The model under review builds one solid part; all positions refer to its coordinate system, in mm. A direction names the side the tool comes from. Round coordinates to 2 decimals unless told otherwise and drop trailing zeros. Order: outer loops, then holes, each group sorted by start corner. A loop starts at its lowest first (then second) coordinate and runs counter-clockwise, first axis right, second up. Notation, with made-up numbers: M -17.5,9 L 22.5,9 A15 ccw 22.5,30 Z; hole C -36,74.25 d4. An arc over 180 degrees is marked long. Use a Markdown table: item, result. Add a question column.
1. Consider section D-D on x = -50.5. State the section outline as (y, z) points, then the cut area to 3 significant figures.
2. To check wall thickness, follow probe 1 along Y at (x, z) = (0, 2.95); probe 2 along Z at (x, y) = (-38.5, -0.25); probe 3 along Y at (x, z) = (-8.5, 12). State the ranges of each line that lie inside material, in increasing order.
3. Consider section C-C on y = 3. State the section outline as (x, z) points, then the cut area to 3 significant figures.
4. Insertion check: P1, Ø4, axis at x = -46, y = -1, coming from the +Z side; P2, Ø1.2, axis at y = -1, z = 10, coming from the +X side; P3, Ø6, axis at x = -41, z = 12.5, coming from the -Y side. Each pin has a flat end and moves straight along its axis. Give the tip position at first contact, or say it passes through.
5. Consider section A-A on x = 0. State the section outline as (y, z) points.
6. The part is to be moulded in two halves that separate along Z. For faces 4 (the flat face through (0, -2, 12.6)), 5 (the flat face through (-33, 0, 6.3)), 6 (the cylindrical face through (-0.37, -1.66, 2.96)), 7 (the flat face through (-4.5, 0, 9)), say which applies: +Z half, -Z half, draft (parallel to the pull), parting line (faces both ways), or undercut.
7. For faces 1 (the flat face through (0, -2, 6)), 2 (the flat face through (-33, 0, 12.3)), 3 (the flat face through (-21, -2, 9)), list the 3-axis set-ups (+Z, -Z, +X, -X, +Y, -Y) from which the entire face can be reached by the end or side of a thin tool; tool diameter is ignored.
8. Consider section B-B on y = 0. State the section outline as (x, z) points.
from build123d import *

# Parameters (mm, degrees)
SKETCH_1_R           = 4
SKETCH_1_R_2         = 1.7
EXTRUDE_1_DEPTH      = 6
EXTRUDE_2_DEPTH      = 2
EXTRUDE_2_DEPTH_BACK = 2
SKETCH_3_R           = 1.7
EXTRUDE_3_DEPTH      = 3
EXTRUDE_3_DEPTH_BACK = 3


with BuildPart() as part:
    # Sketch 1 → Extrude 1 (new body)
    with BuildSketch(Plane.XY):
        Circle(SKETCH_1_R)
        Circle(SKETCH_1_R_2, mode=Mode.SUBTRACT)
    extrude_1 = extrude(amount=EXTRUDE_1_DEPTH)

    # Sketch 2 → Extrude 2 (add, two sides)
    with BuildSketch(Plane(origin=(0, 0, 0), x_dir=(1, 0, 0), z_dir=(0, 1, 0))) as extrude_2_sk:
        Polygon((-4, 0), (-10.5, -6), (-10.5, -12.6), (-4, -18.6), (-3, -18.6), (-3, -12.6), (-4, -12.6), (-4.5, -12.6), (-4.5, -6), (-4, -6), (-3, -6), (-3, 0), align=None)
    extrude(amount=EXTRUDE_2_DEPTH)
    extrude(extrude_2_sk.sketch, amount=-EXTRUDE_2_DEPTH_BACK)

    # Mirror 1: Extrude 1 across plane
    add(extrude_1.mirror(Plane(origin=(0, 0, 9.3), x_dir=(1, 0, 0), z_dir=(0, 0, -1))))

    # Sketch 3 → Extrude 3 (add, two sides)
    with BuildSketch(Plane(origin=(0, 0, 9.3), x_dir=(-1, 0, 0), z_dir=(0, 0, -1))) as extrude_3_sk:
        with BuildLine():
            Line((10.5, 2), (47.035898385, 2))
            ThreePointArc((47.035898385, 2), (54.5, 0), (47.035898385, -2))
            Line((47.035898385, -2), (10.5, -2))
            Line((10.5, -2), (10.5, 2))
        make_face()
        with Locations((50.5, 0)):
            Circle(SKETCH_3_R, mode=Mode.SUBTRACT)
    extrude(amount=EXTRUDE_3_DEPTH)
    extrude(extrude_3_sk.sketch, amount=-EXTRUDE_3_DEPTH_BACK)


solid = part.part
Answer block:
| question | item | result |
|---|---|---|
| 1 | outline | M -4,6.3 L -1.7,6.3 L -1.7,12.3 L -4,12.3 Z; M 1.7,6.3 L 4,6.3 L 4,12.3 L 1.7,12.3 Z |
| 1 | area | 27.6 mm^2 |
| 2 | probe 1 | -4 to -1.7, 1.7 to 4 |
| 2 | probe 2 | 6.3 to 12.3 |
| 2 | probe 3 | -2 to 2 |
| 3 | outline | M -53.15,6.3 L -47.85,6.3 L -47.85,12.3 L -53.15,12.3 Z; M -2.65,0 L 2.65,0 L 2.65,6 L -2.65,6 Z; M -2.65,12.6 L 2.65,12.6 L 2.65,18.6 L -2.65,18.6 Z |
| 3 | area | 95.2 mm^2 |
| 4 | P1 | z = 12.3 |
| 4 | P2 | x = -4.5 |
| 4 | P3 | y = -2 |
| 5 | outline | M -4,0 L -1.7,0 L -1.7,6 L -4,6 Z; M -4,12.6 L -1.7,12.6 L -1.7,18.6 L -4,18.6 Z; M 1.7,0 L 4,0 L 4,6 L 1.7,6 Z; M 1.7,12.6 L 4,12.6 L 4,18.6 L 1.7,18.6 Z |
| 6 | face 4 | undercut |
| 6 | face 5 | -Z half |
| 6 | face 6 | draft |
| 6 | face 7 | undercut |
| 7 | face 1 | +X, +Y, -Y |
| 7 | face 2 | +Z, -X, +Y, -Y |
| 7 | face 3 | +Z, -Z, -Y |
| 8 | outline | M -54.5,6.3 L -52.2,6.3 L -52.2,12.3 L -54.5,12.3 Z; M -48.8,6.3 L -10.5,6.3 L -10.5,6 L -4,0 L -1.7,0 L -1.7,6 L -4.5,6 L -4.5,12.6 L -1.7,12.6 L -1.7,18.6 L -4,18.6 L -10.5,12.6 L -10.5,12.3 L -48.8,12.3 Z; M 1.7,0 L 4,0 L 4,6 L 1.7,6 Z; M 1.7,12.6 L 4,12.6 L 4,18.6 L 1.7,18.6 Z |
